Work out the finished part from the listing and answer in its coordinate system (mm). A direction names the side the tool comes from. Give positions to 0.01 mm unless a question says otherwise; leave off trailing zeros. Loops run counter-clockwise (first coordinate to the right, second up) from the corner with the lowest first, then second, coordinate; pieces in that order, holes last. Notation, with made-up numbers: M 84.25,3 L 106.25,3 A38 ccw 106.25,42 Z; hole C -29,51.5 d4. An arc over 180 degrees is marked long. Write item = value, one per line. Start each with the question number.
1. Section A-A on x = 44 is taken. Give the number of separate pieces and of enclosed holes in the cut face, plus the area to 3 significant figures.
2. Consider L1, parallel to Z at x = 65, y = 6.5; L2, parallel to Z at x = 66.5, y = 12; L3, parallel to X at y = 5.5, z = 4.5 (3 decimals). Determine where each line is inside the solid, lowest interval first. Write a range as [from, to].
3. Flat-ended cylindrical pins translate along their axes: pin 1 Ø2.5 at (x, z) = (37.5, 16) entering from +Y; pin 2 Ø6 at (x, z) = (39.5, -6) entering from +Y; pin 3 Ø2.5 at (x, z) = (37.5, 16.5) entering from -Y. Find the tip coordinate at first contact, or state that the pin passes through.
4. For faces 5 (the face through (27.744, 7, -55)), 6 (the face through (15, 0, 16)), 7 (the face through (20.966, -1.479, -10.965)), 8 (the face through (22.823, -1.521, -19.572)), 9 (the face through (42, 12, 16)), determine the directions among +Z, -Z, +X, -X, +Y, -Y from which every point of the face is accessible in a straight line to the end or side of a thin tool.
5. Section B-B on z = -35 is taken. Determine the outline of the cut face in (x, y), plus the area to 3 significant figures.
6. The mould has two halves that part along Y. Classify faces 1 (the face through (49, 5, -36)), 2 (the face through (20.966, -1.479, -28.965)), 3 (the face through (15, 0, -56)), 4 (the face through (35, 4, 16)): released by +Y, released by -Y, zero draft, split by the parting line, or undercut.
```python
from build123d import *

# Parameters (mm, degrees)
SKETCH2_R           = 2.25
BOSS_EXTRUDE1_DEPTH = 15
SKETCH3_W           = 80
SKETCH3_H           = 37.3
BOSS_EXTRUDE2_DEPTH = 3
SKETCH2_6_W         = 39
SKETCH2_6_H         = 6.4
CUT_EXTRUDE1_DEPTH  = 1
CUT_EXTRUDE4_DEPTH  = 3.1
SKETCH5_W           = 42
SKETCH5_H           = 5
BOSS_EXTRUDE3_DEPTH = 7
SKETCH6_W           = 40.4
SKETCH6_H           = 20.3
CUT_EXTRUDE5_DEPTH  = 0.7
CUT_EXTRUDE6_DEPTH  = 5
SKETCH8_R           = 2.5
CUT_EXTRUDE7_DEPTH  = 5
SKETCH9_R           = 3.25
SKETCH9_R_2         = 1.7
CUT_EXTRUDE8_DEPTH  = 2
SKETCH10_R          = 1.7
CUT_EXTRUDE10_DEPTH = 92.27783365
SKETCH11_R          = 2.25
BOSS_EXTRUDE4_DEPTH = 0.7
SKETCH12_R          = 2.25
BOSS_EXTRUDE5_DEPTH = 0.7
SKETCH13_W          = 80
SKETCH13_H          = 74.6
SKETCH13_R          = 1.7
SKETCH13_W_2        = 5
SKETCH13_H_2        = 10
BOSS_EXTRUDE6_DEPTH = 2
FILLET1_R           = 3
SKETCH14_R          = 3.25
CUT_EXTRUDE11_DEPTH = 1


with BuildPart() as part:
    # Sketch2 → Boss-Extrude1 (new body)
    with BuildSketch(Plane(origin=(0, 0, 0), x_dir=(1, 0, 0), z_dir=(0, 1, 0))):
        Polygon((69.743853574, -17.657592215), (69.743853574, -0.657592215), (27.743853574, -0.657592215), (27.743853574, -8.157592215), (66.743853574, -8.157592215), (66.743853574, -14.557592215), (27.743853574, -14.557592215), (27.743853574, -17.657592215), align=None)
        with Locations(Location((8.493853574, -4.407592215, 0), (0, 0, 270))):
            Circle(SKETCH2_R)
        with BuildLine():
            ThreePointArc((8.493853574, -8.157592215), (5.842203145, -7.059242644), (4.743853574, -4.407592215))
            Line((4.743853574, -4.407592215), (4.743853574, -15.452235072))
            Line((4.743853574, -15.452235072), (8.493853574, -12.907592215))
            Line((8.493853574, -12.907592215), (8.493853574, -8.157592215))
        make_face()
        Polygon((-5.256146426, -0.657592215), (-5.256146426, 19.642407785), (-10.256146426, 19.642407785), (-10.256146426, -17.657592215), (1.493853574, -17.657592215), (4.743853574, -15.452235072), (4.743853574, -4.407592215), (4.743853574, -0.657592215), align=None)
    extrude(amount=BOSS_EXTRUDE1_DEPTH)

    # Sketch3 → Boss-Extrude2 (add)
    with BuildSketch(Plane(origin=(0, 0, 0), x_dir=(-1, 0, 0), z_dir=(0, -1, 0))):
        with Locations((-29.743853574, 0.992407785)):
            Rectangle(SKETCH3_W, SKETCH3_H)
    extrude(amount=BOSS_EXTRUDE2_DEPTH)

    # Sketch2<6> → Cut-Extrude1 (cut)
    with BuildSketch(Plane(origin=(0, 0, 0), x_dir=(1, 0, 0), z_dir=(0, 1, 0))):
        Polygon((27.743853574, -8.157592215), (8.493853574, -8.157592215), (8.493853574, -12.907592215), (8.493853574, -14.557592215), (27.743853574, -14.557592215), align=None)
        with Locations((47.243853574, -11.357592215)):
            Rectangle(SKETCH2_6_W, SKETCH2_6_H)
    extrude(amount=-CUT_EXTRUDE1_DEPTH, mode=Mode.SUBTRACT)

    # Sketch4 → Cut-Extrude4 (cut)
    with BuildSketch(Plane.XY.offset(17.657592215)):
        Polygon((37.543853574, 7), (56.743853574, 7), (56.743853574, 15), (51.743853574, 15), (51.743853574, 12), (32.743853574, 12), (32.743853574, 4), (37.543853574, 4), align=None)
    extrude(amount=-CUT_EXTRUDE4_DEPTH, mode=Mode.SUBTRACT)

    # Sketch5 → Boss-Extrude3 (add)
    with BuildSketch(Plane(origin=(0, 0, 0.657592215), x_dir=(-1, 0, 0), z_dir=(0, 0, -1))):
        with Locations((-48.743853574, 7.5)):
            Rectangle(SKETCH5_W, SKETCH5_H)
    extrude(amount=BOSS_EXTRUDE3_DEPTH)

    # Sketch6 → Cut-Extrude5 (cut)
    with BuildSketch(Plane(origin=(0, 0, 0), x_dir=(1, 0, 0), z_dir=(0, 1, 0))):
        with Locations((49.543853574, 9.492407785)):
            Rectangle(SKETCH6_W, SKETCH6_H)
    extrude(amount=-CUT_EXTRUDE5_DEPTH, mode=Mode.SUBTRACT)

    # Sketch7 → Cut-Extrude6 (cut)
    with BuildSketch(Plane(origin=(0, 0, -19.642407785), x_dir=(-1, 0, 0), z_dir=(0, 0, -1))):
        Polygon((-29.343853574, -0.7), (-26.343853574, -3), (-21.343853574, -3), (-24.343853574, 0), (-29.343853574, 0), align=None)
    extrude(amount=-CUT_EXTRUDE6_DEPTH, mode=Mode.SUBTRACT)

    # Sketch8 → Cut-Extrude7 (cut)
    with BuildSketch(Plane(origin=(0, 15, 0), x_dir=(1, 0, 0), z_dir=(0, 1, 0))):
        with Locations(Location((-2.256146426, -9.657592215, 0), (0, 0, 270))):
            Circle(SKETCH8_R)
        with Locations(Location((59.743853574, -4.407592215, 0), (0, 0, 270))):
            Circle(SKETCH8_R)
    extrude(amount=-CUT_EXTRUDE7_DEPTH, mode=Mode.SUBTRACT)

    # Mirror1: part across plane


with BuildPart() as part_1:
    add(part.part)
    add(part.part.mirror(Plane(origin=(-10.256146426, -3, -19.642407785), x_dir=(1, 0, 0), z_dir=(0, 0, 1))))

    # Sketch9 → Cut-Extrude8 (cut)
    # profile 1 of 3: a face of its own
    with BuildSketch(Plane(origin=(0, 0, 0), x_dir=(1, 0, 0), z_dir=(0, 1, 0))):
        with Locations(Location((17.743853574, 28.542407785, 0), (0, 0, 270))):
            Circle(SKETCH9_R)
        with Locations(Location((17.743853574, 28.542407785, 0), (0, 0, 270))):
            Circle(SKETCH9_R_2, mode=Mode.SUBTRACT)
    # profile 2 of 3: a face of its own
    with BuildSketch(Plane(origin=(0, 0, 0), x_dir=(1, 0, 0), z_dir=(0, 1, 0))):
        with Locations(Location((17.743853574, 10.542407785, 0), (0, 0, 270))):
            Circle(SKETCH9_R)
        with Locations(Location((17.743853574, 10.542407785, 0), (0, 0, 270))):
            Circle(SKETCH9_R_2, mode=Mode.SUBTRACT)
    # profile 3 of 3: a face of its own
    with BuildSketch(Plane(origin=(0, 0, 0), x_dir=(1, 0, 0), z_dir=(0, 1, 0))):
        with Locations(Location((2.743853574, 10.542407785, 0), (0, 0, 270))):
            Circle(SKETCH9_R)
        with Locations(Location((2.743853574, 10.542407785, 0), (0, 0, 270))):
            Circle(SKETCH9_R_2, mode=Mode.SUBTRACT)
    extrude(amount=-CUT_EXTRUDE8_DEPTH, mode=Mode.SUBTRACT)

    # Sketch10 → Cut-Extrude10 (cut, through all)
    with BuildSketch(Plane(origin=(0, 0, 0), x_dir=(1, 0, 0), z_dir=(0, 1, 0))):
        with Locations(Location((17.743853574, 28.542407785, 0), (0, 0, 270))):
            Circle(SKETCH10_R)
        with Locations(Location((17.743853574, 10.542407785, 0), (0, 0, 270))):
            Circle(SKETCH10_R)
        with Locations(Location((2.743853574, 10.542407785, 0), (0, 0, 270))):
            Circle(SKETCH10_R)
    extrude(amount=-CUT_EXTRUDE10_DEPTH, mode=Mode.SUBTRACT)

    # Sketch11 → Boss-Extrude4 (add)
    with BuildSketch(Plane(origin=(0, 15, 0), x_dir=(1, 0, 0), z_dir=(0, 1, 0))):
        with Locations(Location((8.493853574, -4.407592215, 0), (0, 0, 270))):
            Circle(SKETCH11_R)
    extrude(amount=BOSS_EXTRUDE4_DEPTH)

    # Sketch12 → Boss-Extrude5 (add)
    with BuildSketch(Plane(origin=(0, 15, 0), x_dir=(1, 0, 0), z_dir=(0, 1, 0))):
        with Locations(Location((8.493853574, 43.692407785, 0), (0, 0, 270))):
            Circle(SKETCH12_R)
    extrude(amount=BOSS_EXTRUDE5_DEPTH)

    # Sketch13 → Boss-Extrude6 (add)
    with BuildSketch(Plane(origin=(0, -3, 0), x_dir=(-1, 0, 0), z_dir=(0, -1, 0))):
        with Locations((-29.743853574, 19.642407785)):
            Rectangle(SKETCH13_W, SKETCH13_H)
        with Locations(Location((-17.743853574, 28.542407785, 0), (0, 0, 270))):
            Circle(SKETCH13_R, mode=Mode.SUBTRACT)
        with Locations(Location((-17.743853574, 10.542407785, 0), (0, 0, 270))):
            Circle(SKETCH13_R, mode=Mode.SUBTRACT)
        with Locations(Location((-2.743853574, 10.542407785, 0), (0, 0, 270))):
            Circle(SKETCH13_R, mode=Mode.SUBTRACT)
        with Locations((-23.843853574, 19.642407785)):
            Rectangle(SKETCH13_W_2, SKETCH13_H_2, mode=Mode.SUBTRACT)
    extrude(amount=BOSS_EXTRUDE6_DEPTH)

    # Fillet1
    fillet1_edges = [part_1.edges().sort_by_distance(p)[0] for p in [
        (-10.256146426, 5, -56.942407785),
        (-10.256146426, 5, 17.657592215),
        (-10.256146426, -5, -19.642407785),
        (29.743853574, -5, -56.942407785),
        (29.743853574, -5, 17.657592215),
    ]]
    fillet(fillet1_edges, radius=FILLET1_R)

    # Sketch14 → Cut-Extrude11 (cut)
    with BuildSketch(Plane(origin=(0, -2, 0), x_dir=(1, 0, 0), z_dir=(0, 1, 0))):
        with Locations(Location((17.743853574, 28.542407785, 0), (0, 0, 270))):
            Circle(SKETCH14_R)
        with Locations(Location((17.743853574, 10.542407785, 0), (0, 0, 270))):
            Circle(SKETCH14_R)
        with Locations(Location((2.743853574, 10.542407785, 0), (0, 0, 270))):
            Circle(SKETCH14_R)
    extrude(amount=-CUT_EXTRUDE11_DEPTH, mode=Mode.SUBTRACT)


solid = part_1.part
```
Verdict:
q1.separate_pieces = 3
q1.enclosed_holes = 0
q1.area = 685 mm2
q2.L1 = [-56.94, -53.84], [-47.44, -32.94], [-6.34, 8.16], [14.56, 17.66]
q2.L2 = [-56.94, -53.84], [-47.44, -39.94], [0.66, 8.16], [14.56, 17.66]
q2.L3 = [-10.256, 4.745], [6.246, 10.742], [27.744, 69.744]
q3.pin_1 = 15
q3.pin_2 = 10
q3.pin_3 = -4.94
q4.face_5 = +Z, -Z, +Y
q4.face_6 = +Z, +Y
q4.face_7 = +Y
q4.face_8 = -Y
q4.face_9 = +Z
q5.outline = M -10.26,-2 A3 ccw -7.26,-5 L 69.74,-5 L 69.74,-0.7 L 29.34,-0.7 L 29.34,0 L -5.26,0 L -5.26,15 L -10.26,15 Z; M 27.74,5 L 69.74,5 L 69.74,10 L 27.74,10 Z
q5.area = 655 mm2
q6.face_1 = undercut
q6.face_2 = zero draft
q6.face_3 = released by +Y
q6.face_4 = undercut
